Geometry: final body of the model. Coordinates: model frame, mm. A direction names the side the tool comes from. Give positions to 0.01 mm unless a question says otherwise; leave off trailing zeros. Write each loop counter-clockwise with the first axis right and the second up, starting at its lowest first coordinate (ties: lowest second). Pieces come first, ordered by that corner, then holes. Notation, with made-up numbers: M -20.75,-26 L 16.25,-26 A8 cw 16.25,-17 Z; hole C -15,-17 d11. An arc over 180 degrees is marked long. Use a Markdown table: item, result. Add a question column.
(1) Cut plane C-C (z = -69). State how many separate pieces and enclosed holes the cut face has, plus the area to 3 significant figures.
(2) Material intervals for L1, parallel to Y at x = 0.25, z = -8; L2, parallel to X at y = 7, z = -66.5; L3, parallel to X at y = 6.5, z = -57, sorted ascending.
(3) Reachability of faces 5 (the cylindrical face through (-3.25, -11.45, -49.3)), 6 (the flat face through (-7, -12.5, -49)), 7 (the flat face through (0, -4.38, -49)) from +Z, -Z, +X, -X, +Y, -Y: full face, straight path, thin tool, end or side. Return the list, or none.
(4) Draft query along Y for faces 1 (the flat face through (-5, 10.36, -49)), 2 (the flat face through (0, 3, -100)), 3 (the cylindrical face through (-11.935, -11.904, -49.3)), 4 (the cylindrical face through (7.36, 9.73, -49.3)). Return one class per face: released by +Y, released by -Y, zero draft, split by the parting line, or undercut.
(5) Pin query (flat end, axial travel): pin 1 Ø1 at (x, z) = (0, -82.5) entering from +Y; pin 2 Ø0.9 at (x, z) = (0.5, -66.5) entering from -Y; pin 3 Ø1.5 at (x, y) = (-7.5, -5) entering from +Z; pin 4 Ø1 at (x, z) = (-3, -38) entering from +Y. Return the tip coordinate at first contact, or that it passes through.
(6) Cut plane B-B (y = -11.43). Output: boundary loops of the cut face in (x, z).
(7) Cut plane A-A (x = 0). Output: boundary loops of the cut face in (y, z), plus the area to 3 significant figures.
Autodesk Inventor part; units mm, degrees
ref_plane "YZ Plane" through (0, 0, 0) normal (1, 0, 0) x (0, 1, 0)
ref_plane "XZ Plane" through (0, 0, 0) normal (0, 1, 0) x (-1, 0, 0)
ref_plane "XY Plane" through (0, 0, 0) normal (0, 0, 1) x (1, 0, 0)
sketch "Sketch1" plane through (0, 0, 0) normal (0, 0, 1) x (1, 0, 0)
  arc A0 (-10.36, -6.4282) -> (-8.6498, -7.1366) centre (-9.3582, -6.4282) ccw
  line L0 (-10.36, 6.4282) -> (-10.36, -6.4282)
  arc A1 (-8.6498, 7.1366) -> (-10.36, 6.4282) centre (-9.3582, 6.4282) ccw
  line L1 (-5.3093, 3.7961) -> (-8.6498, 7.1366)
  arc A2 (-4.38, 1.5525) -> (-5.3093, 3.7961) centre (-7.553, 1.5525) ccw
  line L2 (-4.38, -1.5525) -> (-4.38, 1.5525)
  arc A3 (-5.3093, -3.7961) -> (-4.38, -1.5525) centre (-7.553, -1.5525) ccw
  line L3 (-8.6498, -7.1366) -> (-5.3093, -3.7961)
  arc A4 (8.6498, -7.1366) -> (10.36, -6.4282) centre (9.3582, -6.4282) ccw
  line L4 (5.3093, -3.7961) -> (8.6498, -7.1366)
  arc A5 (4.38, -1.5525) -> (5.3093, -3.7961) centre (7.553, -1.5525) ccw
  line L5 (4.38, 1.5525) -> (4.38, -1.5525)
  arc A6 (5.3093, 3.7961) -> (4.38, 1.5525) centre (7.553, 1.5525) ccw
  line L6 (8.6498, 7.1366) -> (5.3093, 3.7961)
  arc A7 (10.36, 6.4282) -> (8.6498, 7.1366) centre (9.3582, 6.4282) ccw
  line L7 (10.36, -6.4282) -> (10.36, 6.4282)
  circle A8 centre (0, 0) radius 2.5
  line L8 (-10.5183, -12.5) -> (-4.32, -12.5)
  arc A9 (-4.32, -12.5) -> (-4.32, -10.36) centre (-4.32, -11.43) ccw
  line L9 (-4.32, -10.36) -> (-6.4282, -10.36)
  arc A10 (-7.1366, -8.6498) -> (-6.4282, -10.36) centre (-6.4282, -9.3582) ccw
  line L10 (-7.1366, -8.6498) -> (-3.7961, -5.3093)
  arc A11 (-1.5525, -4.38) -> (-3.7961, -5.3093) centre (-1.5525, -7.553) ccw
  line L11 (-1.5525, -4.38) -> (1.5525, -4.38)
  arc A12 (3.7961, -5.3093) -> (1.5525, -4.38) centre (1.5525, -7.553) ccw
  line L12 (3.7961, -5.3093) -> (7.1366, -8.6498)
  arc A13 (6.4282, -10.36) -> (7.1366, -8.6498) centre (6.4282, -9.3582) ccw
  line L13 (6.4282, -10.36) -> (4.32, -10.36)
  arc A14 (4.32, -10.36) -> (4.32, -12.5) centre (4.32, -11.43) ccw
  line L14 (4.32, -12.5) -> (10.5183, -12.5)
  arc A15 (10.5183, -12.5) -> (12.5, -10.5183) centre (10.5183, -10.5183) ccw
  line L15 (12.5, -10.5183) -> (12.5, 10.5183)
  arc A16 (12.5, 10.5183) -> (10.5183, 12.5) centre (10.5183, 10.5183) ccw
  line L16 (10.5183, 12.5) -> (4.32, 12.5)
  arc A17 (4.32, 12.5) -> (4.32, 10.36) centre (4.32, 11.43) ccw
  line L17 (4.32, 10.36) -> (6.4282, 10.36)
  arc A18 (7.1366, 8.6498) -> (6.4282, 10.36) centre (6.4282, 9.3582) ccw
  line L18 (7.1366, 8.6498) -> (3.7961, 5.3093)
  arc A19 (1.5525, 4.38) -> (3.7961, 5.3093) centre (1.5525, 7.553) ccw
  line L19 (1.5525, 4.38) -> (-1.5525, 4.38)
  arc A20 (-3.7961, 5.3093) -> (-1.5525, 4.38) centre (-1.5525, 7.553) ccw
  line L20 (-3.7961, 5.3093) -> (-7.1366, 8.6498)
  arc A21 (-6.4282, 10.36) -> (-7.1366, 8.6498) centre (-6.4282, 9.3582) ccw
  line L21 (-6.4282, 10.36) -> (-4.32, 10.36)
  arc A22 (-4.32, 10.36) -> (-4.32, 12.5) centre (-4.32, 11.43) ccw
  line L22 (-4.32, 12.5) -> (-10.5183, 12.5)
  arc A23 (-10.5183, 12.5) -> (-12.5, 10.5183) centre (-10.5183, 10.5183) ccw
  line L23 (-12.5, 10.5183) -> (-12.5, -10.5183)
  arc A24 (-12.5, -10.5183) -> (-10.5183, -12.5) centre (-10.5183, -10.5183) ccw
extrude "Extrusion1" add sketch "Sketch1" against normal blind 100
properties part number "25-2504"
Answer list:
| question | item | result |
|---|---|---|
| 1 | separate pieces | 1 |
| 1 | enclosed holes | 3 |
| 1 | area | 304 mm² |
| 2 | L1 | -4.38 to -2.49, 2.49 to 4.38 |
| 2 | L2 | -12.5 to -10.18, -8.51 to -5.49, 5.49 to 8.51, 10.18 to 12.5 |
| 2 | L3 | -12.5 to -10.36, -8.01 to -4.99, 4.99 to 8.01, 10.36 to 12.5 |
| 3 | face 5 | +Z, -Z |
| 3 | face 6 | +Z, -Z, +X, -X, -Y |
| 3 | face 7 | +Z, -Z, -Y |
| 4 | face 1 | undercut |
| 4 | face 2 | zero draft |
| 4 | face 3 | released by -Y |
| 4 | face 4 | undercut |
| 5 | pin 1 | y = 4.38 |
| 5 | pin 2 | y = -4.38 |
| 5 | pin 3 | z = 0 |
| 5 | pin 4 | y = 12.12 |
| 6 | outline | M -12.28,-100 L -3.25,-100 L -3.25,0 L -12.28,0 Z; M 3.25,-100 L 12.28,-100 L 12.28,0 L 3.25,0 Z |
| 7 | outline | M -4.38,-100 L -2.5,-100 L -2.5,0 L -4.38,0 Z; M 2.5,-100 L 4.38,-100 L 4.38,0 L 2.5,0 Z |
| 7 | area | 376 mm² |
